Geometry check sheet. Reference: the model listing, model coordinates, mm. A direction names the side the tool comes from. Give positions to 0.01 mm unless a question says otherwise; leave off trailing zeros. Write each loop counter-clockwise with the first axis right and the second up, starting at its lowest first coordinate (ties: lowest second). Pieces come first, ordered by that corner, then holes. Notation, with made-up numbers: (15.25, -11) - (63.25, -11) arc R28 cw to (63.25, 10) - close; hole circle Ø3 at (42.5, 6.25). An arc over 180 degrees is marked (long way). Write item = value, one per line. Start each with the question number.
(1) Access from +Z, -Z, +X, -X, +Y, -Y to the whole of each face (thin tool, end or side, straight path). Record for faces 1 (the cylindrical face through (-29.062, 15.178, 0.74)), 2 (the flat face through (20.12, -23.264, 0.74)).
(2) Thickness scan on L1, parallel to Y at x = 22.5, z = 0.6 (3 decimals); L2, parallel to Y at x = -24.5, z = 0.85 (3 decimals); L3, parallel to X at y = -6, z = 0.3. Record the ranges inside material, lowest first.
(3) Section check A-A, the plane x = 10. Enter the section's corners in (y, z) (3 decimals).
(4) Depth check by flat-ended pin: pin 1 Ø2.5 at (x, y) = (15.25, -15.25) entering from -Z. Enter the tip coordinate at first touch or a pass-through.
(5) Section check B-B, the plane z = 0.45. Give the number of separate pieces and of enclosed holes in the cut face, plus the area to 3 significant figures.
```python
from build123d import *

# Parameters (mm, degrees)
F0_R     = 1.5
F1_DEPTH = 1.5


with BuildPart() as f1:
    # F0 (on Top) → F1 (new body)
    with BuildSketch(Plane.XY):
        with BuildLine():
            ThreePointArc((26, 0), (29.003525, 14.971686), (34.274381, 29.303142))
            ThreePointArc((34.274381, 29.303142), (34.556043, 31.528729), (33.516861, 33.516861))
            ThreePointArc((33.516861, 33.516861), (31.528729, 34.556043), (29.303142, 34.274381))
            ThreePointArc((29.303142, 34.274381), (14.971686, 29.003525), (0, 26))
            ThreePointArc((0, 26), (-14.971686, 29.003525), (-29.303142, 34.274381))
            ThreePointArc((-29.303142, 34.274381), (-31.528729, 34.556043), (-33.516861, 33.516861))
            ThreePointArc((-33.516861, 33.516861), (-34.556043, 31.528729), (-34.274381, 29.303142))
            ThreePointArc((-34.274381, 29.303142), (-29.003525, 14.971686), (-26, 0))
            ThreePointArc((-26, 0), (-29.003525, -14.971686), (-34.274381, -29.303142))
            ThreePointArc((-34.274381, -29.303142), (-34.556043, -31.528729), (-33.516861, -33.516861))
            ThreePointArc((-33.516861, -33.516861), (-31.590724, -34.544359), (-29.418712, -34.325))
            Line((-29.418712, -34.325), (29.418712, -34.325))
            ThreePointArc((29.418712, -34.325), (31.590724, -34.544359), (33.516861, -33.516861))
            ThreePointArc((33.516861, -33.516861), (34.556043, -31.528729), (34.274381, -29.303142))
            ThreePointArc((34.274381, -29.303142), (29.003525, -14.971686), (26, 0))
        make_face()
        with Locations((-29.392136, -29.392136)):
            Circle(F0_R, mode=Mode.SUBTRACT)
        with BuildLine():
            ThreePointArc((-24.324473, -24.324473), (-24.671832, -23.656327), (-24.572337, -22.909884))
            Line((-24.572337, -22.909884), (-21.918806, -17.251149))
            ThreePointArc((-21.918806, -17.251149), (-20.871666, -16.534722), (-19.73736, -17.103157))
            Line((-19.73736, -17.103157), (-18.702974, -18.702974))
            Line((-18.702974, -18.702974), (-17.103157, -19.73736))
            ThreePointArc((-17.103157, -19.73736), (-16.534722, -20.871666), (-17.251149, -21.918806))
            Line((-17.251149, -21.918806), (-22.909884, -24.572337))
            ThreePointArc((-22.909884, -24.572337), (-23.656327, -24.671832), (-24.324473, -24.324473))
        make_face(mode=Mode.SUBTRACT)
        with BuildLine():
            Line((-11, -27.025), (-5, -27.025))
            ThreePointArc((-5, -27.025), (-4, -28.025), (-5, -29.025))
            Line((-5, -29.025), (-11, -29.025))
            ThreePointArc((-11, -29.025), (-12, -28.025), (-11, -27.025))
        make_face(mode=Mode.SUBTRACT)
        with Locations((-15.25, -15.25)):
            Circle(F0_R, mode=Mode.SUBTRACT)
        with Locations((0, -28.025)):
            Circle(F0_R, mode=Mode.SUBTRACT)
        with BuildLine():
            ThreePointArc((5, -29.025), (4, -28.025), (5, -27.025))
            Line((5, -27.025), (11, -27.025))
            ThreePointArc((11, -27.025), (12, -28.025), (11, -29.025))
            Line((11, -29.025), (5, -29.025))
        make_face(mode=Mode.SUBTRACT)
        with Locations((29.392136, -29.392136)):
            Circle(F0_R, mode=Mode.SUBTRACT)
        with BuildLine():
            Line((21.918806, -17.251149), (24.572337, -22.909884))
            ThreePointArc((24.572337, -22.909884), (24.671832, -23.656327), (24.324473, -24.324473))
            ThreePointArc((24.324473, -24.324473), (23.656327, -24.671832), (22.909884, -24.572337))
            Line((22.909884, -24.572337), (17.251149, -21.918806))
            ThreePointArc((17.251149, -21.918806), (16.534722, -20.871666), (17.103157, -19.73736))
            Line((17.103157, -19.73736), (18.702974, -18.702974))
            Line((18.702974, -18.702974), (19.73736, -17.103157))
            ThreePointArc((19.73736, -17.103157), (20.871666, -16.534722), (21.918806, -17.251149))
        make_face(mode=Mode.SUBTRACT)
        with BuildLine():
            ThreePointArc((8.383883, -15.31353), (8.608023, -16.776019), (7.279787, -17.427863))
            Line((7.279787, -17.427863), (0, -16.125))
            Line((0, -16.125), (-7.279787, -17.427863))
            ThreePointArc((-7.279787, -17.427863), (-8.608023, -16.776019), (-8.383883, -15.31353))
            Line((-8.383883, -15.31353), (-0.883883, -7.81353))
            ThreePointArc((-0.883883, -7.81353), (0, -7.447413), (0.883883, -7.81353))
            Line((0.883883, -7.81353), (8.383883, -15.31353))
        make_face(mode=Mode.SUBTRACT)
        with Locations((15.25, -15.25)):
            Circle(F0_R, mode=Mode.SUBTRACT)
        with BuildLine():
            Line((-16.125, 0), (-17.427863, 7.279787))
            ThreePointArc((-17.427863, 7.279787), (-16.776019, 8.608023), (-15.31353, 8.383883))
            Line((-15.31353, 8.383883), (-7.81353, 0.883883))
            ThreePointArc((-7.81353, 0.883883), (-7.447413, 0), (-7.81353, -0.883883))
            Line((-7.81353, -0.883883), (-15.31353, -8.383883))
            ThreePointArc((-15.31353, -8.383883), (-16.776019, -8.608023), (-17.427863, -7.279787))
            Line((-17.427863, -7.279787), (-16.125, 0))
        make_face(mode=Mode.SUBTRACT)
        with Locations((-15.25, 15.25)):
            Circle(F0_R, mode=Mode.SUBTRACT)
        with BuildLine():
            ThreePointArc((-17.251149, 21.918806), (-16.534722, 20.871666), (-17.103157, 19.73736))
            Line((-17.103157, 19.73736), (-18.702974, 18.702974))
            Line((-18.702974, 18.702974), (-19.73736, 17.103157))
            ThreePointArc((-19.73736, 17.103157), (-20.871666, 16.534722), (-21.918806, 17.251149))
            Line((-21.918806, 17.251149), (-24.572337, 22.909884))
            ThreePointArc((-24.572337, 22.909884), (-24.671832, 23.656327), (-24.324473, 24.324473))
            ThreePointArc((-24.324473, 24.324473), (-23.656327, 24.671832), (-22.909884, 24.572337))
            Line((-22.909884, 24.572337), (-17.251149, 21.918806))
        make_face(mode=Mode.SUBTRACT)
        with Locations((-29.392136, 29.392136)):
            Circle(F0_R, mode=Mode.SUBTRACT)
        with BuildLine():
            ThreePointArc((7.81353, -0.883883), (7.447413, 0), (7.81353, 0.883883))
            Line((7.81353, 0.883883), (15.31353, 8.383883))
            ThreePointArc((15.31353, 8.383883), (16.776019, 8.608023), (17.427863, 7.279787))
            Line((17.427863, 7.279787), (16.125, 0))
            Line((16.125, 0), (17.427863, -7.279787))
            ThreePointArc((17.427863, -7.279787), (16.776019, -8.608023), (15.31353, -8.383883))
            Line((15.31353, -8.383883), (7.81353, -0.883883))
        make_face(mode=Mode.SUBTRACT)
        with BuildLine():
            Line((-7.279787, 17.427863), (0, 16.125))
            Line((0, 16.125), (7.279787, 17.427863))
            ThreePointArc((7.279787, 17.427863), (8.608023, 16.776019), (8.383883, 15.31353))
            Line((8.383883, 15.31353), (0.883883, 7.81353))
            ThreePointArc((0.883883, 7.81353), (0, 7.447413), (-0.883883, 7.81353))
            Line((-0.883883, 7.81353), (-8.383883, 15.31353))
            ThreePointArc((-8.383883, 15.31353), (-8.608023, 16.776019), (-7.279787, 17.427863))
        make_face(mode=Mode.SUBTRACT)
        with Locations((15.25, 15.25)):
            Circle(F0_R, mode=Mode.SUBTRACT)
        with BuildLine():
            Line((19.73736, 17.103157), (18.702974, 18.702974))
            Line((18.702974, 18.702974), (17.103157, 19.73736))
            ThreePointArc((17.103157, 19.73736), (16.534722, 20.871666), (17.251149, 21.918806))
            Line((17.251149, 21.918806), (22.909884, 24.572337))
            ThreePointArc((22.909884, 24.572337), (23.656327, 24.671832), (24.324473, 24.324473))
            ThreePointArc((24.324473, 24.324473), (24.671832, 23.656327), (24.572337, 22.909884))
            Line((24.572337, 22.909884), (21.918806, 17.251149))
            ThreePointArc((21.918806, 17.251149), (20.871666, 16.534722), (19.73736, 17.103157))
        make_face(mode=Mode.SUBTRACT)
        with Locations((29.392136, 29.392136)):
            Circle(F0_R, mode=Mode.SUBTRACT)
    extrude(amount=F1_DEPTH)


solid = f1.part
```
Model answer:
q1.face_1 = +Z, -Z, -X
q1.face_2 = +Z, -Z
q2.L1 = -34.325 to -24.38, -18.491 to 18.491, 24.38 to 31.458
q2.L2 = -34.325 to -24.104, -22.756 to 22.756, 24.104 to 32.225
q2.L3 = -26.92 to -17.2, -12.93 to 12.93, 17.2 to 26.92
q3.outline = (-34.325, 0) - (-29.025, 0) - (-29.025, 1.5) - (-34.325, 1.5) - close; (-27.025, 0) - (-3.07, 0) - (-3.07, 1.5) - (-27.025, 1.5) - close; (3.07, 0) - (27.738, 0) - (27.738, 1.5) - (3.07, 1.5) - close
q4.pin_1 = through
q5.separate_pieces = 1
q5.enclosed_holes = 19
q5.area = 3,200 mm²
